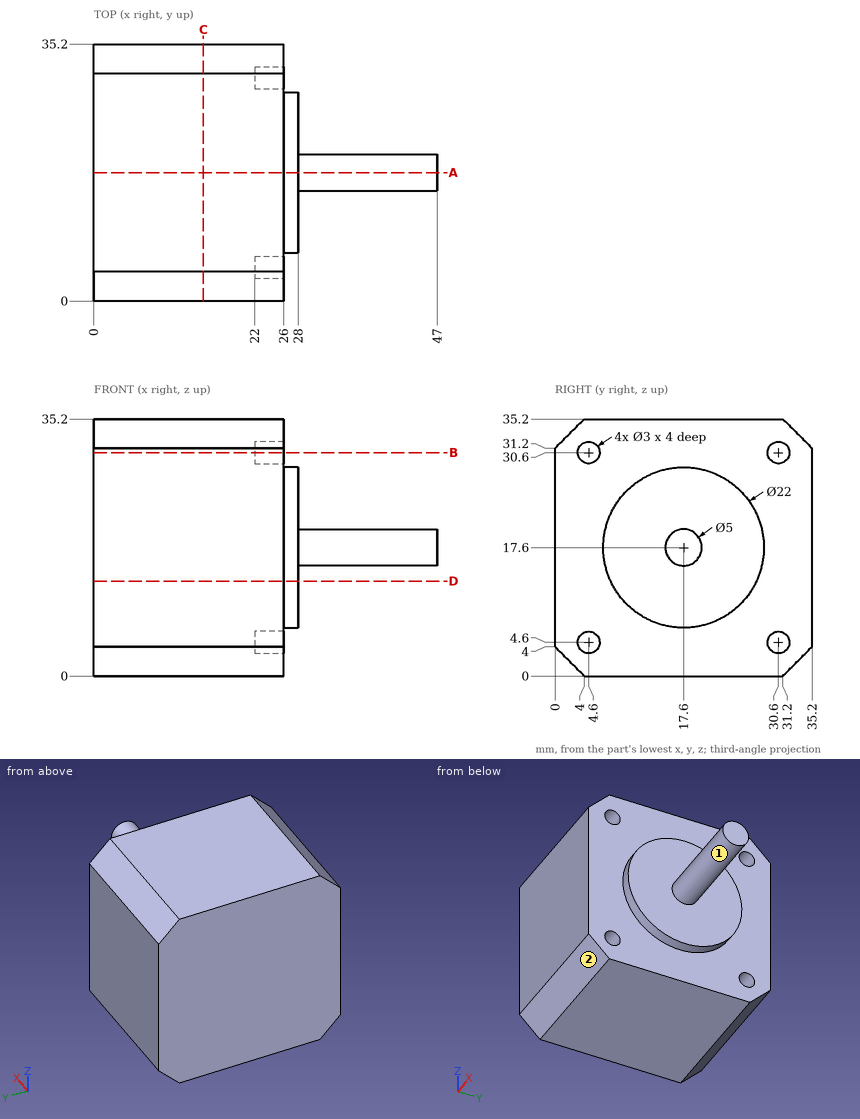
Verification items for this drawing (mm, ordinates from the low corner). A direction names the side the tool comes from. Give positions to 0.01 mm unless a question says otherwise; leave off trailing zeros. Loops run counter-clockwise (first coordinate to the right, second up) from the corner with the lowest first, then second, coordinate; pieces in that order, holes last. Notation, with made-up numbers: M 46,-7 L 77,-7 A30 cw 77,15 Z; hole C -38,-22.5 d5. An arc over 180 degrees is marked long. Answer in a Markdown table with one row per item.
1) Thickness scan on line 1 (Y direction, x = 23, z = 30.6); line 2 (Y direction, x = 24, z = 30); line 3 (X direction, y = 21.5, z = 10). Record the ranges inside material, lowest first.
Solutions:
| item | result |
|---|---|
| line 1 | y = 0 to 3.1, 6.1 to 29.1, 32.1 to 35.2 |
| line 2 | y = 0 to 3.23, 5.97 to 29.23, 31.97 to 35.2 |
| line 3 | x = 0 to 28 |
2) Cross-section at B-B (z = 30.6). Enter the section's corners in (x, y), plus the area to 3 significant figures.
Solutions:
| item | result |
|---|---|
| outline | M 0,0 L 26,0 L 26,3.1 L 22,3.1 L 22,6.1 L 26,6.1 L 26,29.1 L 22,29.1 L 22,32.1 L 26,32.1 L 26,35.2 L 0,35.2 Z |
| area | 891 mm^2 |
3) Cross-section at A-A (y = 17.6). Enter the section's corners in (x, z).
Solutions:
| item | result |
|---|---|
| outline | M 0,0 L 26,0 L 26,6.6 L 28,6.6 L 28,15.1 L 47,15.1 L 47,20.1 L 28,20.1 L 28,28.6 L 26,28.6 L 26,35.2 L 0,35.2 Z |
4) Tool access check on the marked faces 1 and 2. Record the directions out of +Z, -Z, +X, -X, +Y, -Y that give a thin tool (end or side, any length) a straight path to the whole face; none if there is none.
Solutions:
| item | result |
|---|---|
| face 1 | +X |
| face 2 | -Z, +X, -X, -Y |
5) Cross-section at C-C (x = 15). Enter the section's corners in (y, z), plus the area to 3 significant figures.
Solutions:
| item | result |
|---|---|
| outline | M 0,4 L 4,0 L 31.2,0 L 35.2,4 L 35.2,31.2 L 31.2,35.2 L 4,35.2 L 0,31.2 Z |
| area | 1,210 mm^2 |
6) Cross-section at D-D (z = 13). Enter the section's corners in (x, y), plus the area to 3 significant figures.
Solutions:
| item | result |
|---|---|
| outline | M 0,0 L 26,0 L 26,7.61 L 28,7.61 L 28,27.59 L 26,27.59 L 26,35.2 L 0,35.2 Z |
| area | 955 mm^2 |
7) Depth check by flat-ended pin: pin 1 (1.5 mm diameter, centred on y = 4, z = 4.5, fed in from +X); pin 2 (2.5 mm diameter, centred on y = 30, z = 31, fed in from +X); pin 3 (12 mm diameter, centred on x = 39, z = 19.5, fed in from +Y). Enter the tip coordinate at first touch or a pass-through.
Solutions:
| item | result |
|---|---|
| pin 1 | stops at x = 22 |
| pin 2 | stops at x = 26 |
| pin 3 | stops at y = 20.1 |
